Read the model definition and answer for the solid it produces. Units are mm, in the model's axes. A direction names the side the tool comes from. Give positions to 0.01 mm unless a question says otherwise; leave off trailing zeros. Order: outer loops, then holes, each group sorted by start corner. A loop starts at its lowest first (then second) coordinate and runs counter-clockwise, first axis right, second up.
```python
from build123d import *

# Parameters (mm, degrees)
F0_W      = 450
F0_H      = 200
F1_DEPTH  = 9
F2_W      = 4.5
F2_H      = 200
F3_DEPTH  = 4.5
F4_W      = 4.5
F4_H      = 200
F5_DEPTH  = 4.5
F6_W      = 441
F6_H      = 4.5
F7_DEPTH  = 4.5
F8_W      = 395
F8_H      = 121
F9_DEPTH  = 9
F10_R     = 2.5
F11_DEPTH = 9


with BuildPart() as f1:
    # F0 (on Right) → F1 (new body)
    with BuildSketch(Plane.YZ):
        Rectangle(F0_W, F0_H)
    extrude(amount=F1_DEPTH)

    # F2 (on face) → F3 (cut)
    with BuildSketch(Plane.XZ.offset(225)):
        with Locations((2.25, 0)):
            Rectangle(F2_W, F2_H)
    extrude(amount=-F3_DEPTH, mode=Mode.SUBTRACT)

    # F4 (on face) → F5 (cut)
    with BuildSketch(Plane(origin=(0, 225, 0), x_dir=(-1, 0, 0), z_dir=(0, 1, 0))):
        with Locations((-2.25, 0)):
            Rectangle(F4_W, F4_H)
    extrude(amount=-F5_DEPTH, mode=Mode.SUBTRACT)

    # F6 (on face) → F7 (cut)
    with BuildSketch(Plane(origin=(0, 0, 0), x_dir=(0, -1, 0), z_dir=(-1, 0, 0))):
        with Locations((0, -52.75)):
            Rectangle(F6_W, F6_H)
    extrude(amount=-F7_DEPTH, mode=Mode.SUBTRACT)

    # F8 (on face) → F9 (cut, through all)
    with BuildSketch(Plane.YZ.offset(9)):
        with Locations((8, 14.5)):
            Rectangle(F8_W, F8_H)
    extrude(amount=-F9_DEPTH, mode=Mode.SUBTRACT)

    # F10 (on face) → F11 (cut, through all)
    with BuildSketch(Plane.YZ.offset(9)):
        with Locations((203.5, 84)):
            Circle(F10_R)
        with Locations((-171.5, 84)):
            Circle(F10_R)
        with Locations((-171.5, -55)):
            Circle(F10_R)
        with Locations((203.5, -55)):
            Circle(F10_R)
    extrude(amount=-F11_DEPTH, mode=Mode.SUBTRACT)


solid = f1.part
```
1) For a pull along Y with two mould halves and no side action, classify faces 1 (the face through (5, 5, 75)), 2 (the face through (0, -17.4, 75.3)) as released by +Y, released by -Y, zero draft, split by the parting line, or undercut.
Final values:
face 1: undercut
face 2: zero draft
2) The part is cut by section B-B on y = -97.5. Determine the outline of the cut face in (x, z), and give its area (3 significant figures).
Final values:
outline: (0, -100) - (9, -100) - (9, -46) - (0, -46) - (0, -50.5) - (4.5, -50.5) - (4.5, -55) - (0, -55) - close; (0, 75) - (9, 75) - (9, 100) - (0, 100) - close
area: 691 mm2
3) Given pin 1 (5 mm diameter, centred on x = 1.5, z = 40, fed in from -Y); pin 2 (2 mm diameter, centred on x = 2, z = -86.5, fed in from +Y); pin 3 (6 mm diameter, centred on y = -171.5, z = 84, fed in from +X), each flat-ended and moving along its own axis, determine where each tip first touches the part or whether it passes through.
Final values:
pin 1: stops at y = -220.5
pin 2: stops at y = 220.5
pin 3: stops at x = 9
4) Consider L1, parallel to Z at x = 7, y = 203.5; L2, parallel to Z at x = 2, y = 121; L3, parallel to Y at x = 2.75, z = -4.5. Determine where each line is inside the solid, lowest interval first.
Final values:
L1: z = -100 to -57.5, -52.5 to -46, 75 to 81.5, 86.5 to 100
L2: z = -100 to -55, -50.5 to -46, 75 to 100
L3: y = -220.5 to -189.5, 205.5 to 220.5
5) A tool of negligible diameter and unlimited length cuts with its end or side. For faces 3 (the face through (9, -53, -65)), 4 (the face through (5, 5, -46)), from which of +Z, -Z, +X, -X, +Y, -Y can it reach the whole face along a straight path? Write none if from no direction.
Final values:
face 3: +Z, -Z, +X, +Y, -Y
face 4: +X, -X
6) The part is cut by section A-A on x = 3. Determine the outline of the cut face in (y, z).
Final values:
outline: (-220.5, -100) - (220.5, -100) - (220.5, -55) - (206, -55) arc R2.5 cw to (201, -55) - (-169, -55) arc R2.5 cw to (-174, -55) - (-220.5, -55) - close; (-220.5, -50.5) - (220.5, -50.5) - (220.5, 100) - (-220.5, 100) - close; hole (-189.5, -46) - (205.5, -46) - (205.5, 75) - (-189.5, 75) - close; hole circle Ø5 at (-171.5, 84); hole circle Ø5 at (203.5, 84)
